```python
from build123d import *

# Parameters (mm, degrees)
SKETCH1_R           = 17
SKETCH1_R_2         = 8
BOSS_EXTRUDE4_DEPTH = 2
REVOLVE2_ANGLE      = 40
CIRPATTERN1_COUNT   = 3
FILLET1_R           = 5
BOSS_EXTRUDE6_DEPTH = 13
FILLET2_R           = 0.25
SKETCH25_R          = 0.9
CUT_EXTRUDE1_DEPTH  = 34.719430639
SKETCH26_R          = 1.55
CUT_EXTRUDE2_DEPTH  = 0.8


with BuildPart() as part:
    # Sketch1 → Boss-Extrude4 (new body)
    with BuildSketch(Plane(origin=(0, 0, 0), x_dir=(1, 0, 0), z_dir=(0, 1, 0))):
        with Locations(Location((0, 0, 0), (0, 0, 270))):
            Circle(SKETCH1_R)
        with Locations(Location((0, 0, 0), (0, 0, 270))):
            Circle(SKETCH1_R_2, mode=Mode.SUBTRACT)
    extrude(amount=BOSS_EXTRUDE4_DEPTH)

    # Sketch5 → Revolve2 (revolve)
    with BuildSketch(Plane.XY):
        Polygon((-17, 0), (-22, 0), (-21, 14), (-17, 14), align=None)
    revolve2 = revolve(axis=Axis((0, 9.813682869, 0), (0, -1, 0)), revolution_arc=REVOLVE2_ANGLE)

    # CirPattern1: Revolve2 ×3 about axis
    cirpattern1_axis = Axis((0, 0, 0), (0, 1, 0))
    for i in range(1, CIRPATTERN1_COUNT):
        add(revolve2.rotate(cirpattern1_axis, i * 360 / CIRPATTERN1_COUNT))

    # Fillet1
    fillet1_edges = [part.edges().sort_by_distance(p)[0] for p in [
        (-13.022755533, 1, -10.927389365),
        (-17, 1, 0),
        (-2.95201902, 1, 16.741731801),
        (8.5, 1, 14.722431864),
        (15.974774553, 1, -5.814342437),
        (8.5, 1, -14.722431864),
    ]]
    fillet(fillet1_edges, radius=FILLET1_R)

    # Sketch24 → Boss-Extrude6 (add)
    with BuildSketch(Plane(origin=(0, 2, 0), x_dir=(1, 0, 0), z_dir=(0, 1, 0))):
        with BuildLine():
            ThreePointArc((12.528097784, 11.491160338), (12.448209945, 10.445288373), (13.492065142, 10.342348776))
            ThreePointArc((13.492065142, 10.342348776), (13.022755533, 10.927389365), (12.528097784, 11.491160338))
        make_face()
    extrude(amount=BOSS_EXTRUDE6_DEPTH)

    # Fillet2
    # the kernel refuses this fillet: 0.25 mm, written as the material it takes off along each edge
    with BuildSketch(Plane(origin=(0, 15, 0), x_dir=(0.8154762444384231, 0, -0.578790544805809), z_dir=(0.578790544805809, 0, 0.8154762444384231))) as fillet2_piece_1:
        with BuildLine():
            CenterArc((17 - FILLET2_R, -FILLET2_R), FILLET2_R, 0, 90)
            Line((17 - FILLET2_R, 0), (17, 0))
            Line((17, 0), (17, -FILLET2_R))
        make_face()
    revolve(axis=Axis((0, 15, 0), (0, 1, 0)), revolution_arc=9.268958216, mode=Mode.SUBTRACT)

    # Sketch25 → Cut-Extrude1 (cut, through all)
    with BuildSketch(Plane(origin=(0, 2, 0), x_dir=(1, 0, 0), z_dir=(0, 1, 0))):
        with Locations(Location((2.083778132, -11.817693036, 0), (0, 0, 270))):
            Circle(SKETCH25_R)
        with Locations(Location((-11.236091343, 4.089602798, 0), (0, 0, 270))):
            Circle(SKETCH25_R)
        with Locations(Location((9.192533317, 7.713451316, 0), (0, 0, 270))):
            Circle(SKETCH25_R)
    extrude(amount=-CUT_EXTRUDE1_DEPTH, mode=Mode.SUBTRACT)

    # Sketch26 → Cut-Extrude2 (cut)
    with BuildSketch(Plane(origin=(0, 2, 0), x_dir=(1, 0, 0), z_dir=(0, 1, 0))):
        with Locations(Location((2.083778132, -11.817693036, 0), (0, 0, 270))):
            Circle(SKETCH26_R)
        with Locations(Location((-11.236091343, 4.089602798, 0), (0, 0, 270))):
            Circle(SKETCH26_R)
        with Locations(Location((9.192533317, 7.713451316, 0), (0, 0, 270))):
            Circle(SKETCH26_R)
    extrude(amount=-CUT_EXTRUDE2_DEPTH, mode=Mode.SUBTRACT)


solid = part.part
```
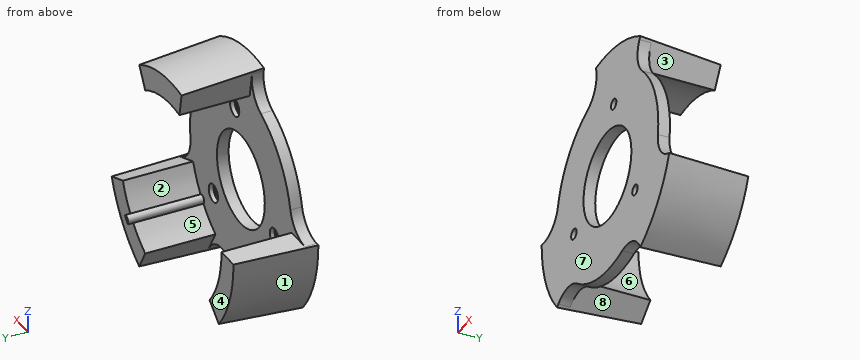
Geometry check sheet. Reference: the model listing, model coordinates, mm. Face numbers are marked on the shaded views. A direction names the side the tool comes from. Coordinates: 2 decimals unless noted, no trailing zeros. Loops run counter-clockwise (first coordinate to the right, second up) from the corner with the lowest first, then second, coordinate; pieces in that order, holes last. Notation, with made-up numbers: (-22, 42.5) - (4, 42.5) arc R16 cw to (4, 66.5) - close; hole circle Ø2 at (-11.5, 32.5). An arc over 180 degrees is marked (long way). One line per item, written item: value. Start each with the question number.
(1) Cross-section at D-D on y = 4. Enter the section's corners in (x, z).
(2) Mould release check, pull along Z, two halves, no side actions. Record for the marked faces 1, 2, 3 and 4: released by +Z, released by -Z, zero draft, split by the parting line, or undercut.
(3) Tool access check on the marked faces 5, 6, 7 and 8. Record the directions out of +Z, -Z, +X, -X, +Y, -Y that give a thin tool (end or side, any length) a straight path to the whole face; none if there is none.
(4) Material ranges on line 1 (Z direction, x = 1, y = 1.5); line 2 (Y direction, x = -8, z = -12.5); line 3 (Y direction, x = 18.5, z = -9.5), recorded low to high. Write a range as [from, to].
(5) Cross-section at B-B on y = 10.75. Enter the section's corners in (x, z).
(6) Cross-section at A-A on x = 0. Enter the section's corners in (y, z).
(7) Depth check by flat-ended pin: P1, Ø5, axis at x = 1.5, y = 8.5, coming from the -Z side; P2, Ø3, axis at x = 2, z = 17, coming from the +Y side; P3, Ø4, axis at x = -10, z = 16, coming from the +Y side. Enter the tip coordinate at first touch or a pass-through.
(8) Cross-section at C-C on x = -15.5. Enter the section's corners in (y, z).
Results below:
1. outline: (-21.71, 0) arc R21.71 ccw to (-16.63, -13.96) - (-13.02, -10.93) arc R17 cw to (-17, 0) - close; (-3.77, 21.38) - (-2.95, 16.74) arc R17 cw to (8.5, 14.72) - (10.86, 18.81) arc R21.71 ccw to start; (8.5, -14.72) - (10.86, -18.81) arc R21.71 ccw to (20.4, -7.43) - (15.97, -5.81) arc R17 cw to (13.49, -10.34) arc R0.75 ccw to (12.53, -11.49) arc R17 cw to start
2. face 1: released by -Z
2. face 2: released by +Z
2. face 3: undercut
2. face 4: zero draft
3. face 5: +Y
3. face 6: +Z, +Y
3. face 7: +Z, -Z, +X, -X, -Y
3. face 8: -Z, +Y
4. line 1: z = [-16.97, -7.94], [7.94, 10.71], [12.93, 21.87]
4. line 2: y = [0, 2]
4. line 3: y = [0, 14]
5. outline: (-21.23, 0) arc R21.23 ccw to (-16.26, -13.65) - (-13.02, -10.93) arc R17 cw to (-17, 0) - close; (-3.69, 20.91) - (-2.95, 16.74) arc R17 cw to (8.5, 14.72) - (10.62, 18.39) arc R21.23 ccw to start; (8.5, -14.72) - (10.62, -18.39) arc R21.23 ccw to (19.95, -7.26) - (15.97, -5.81) arc R17 cw to (13.49, -10.34) arc R0.75 ccw to (12.53, -11.49) arc R17 cw to start
6. outline: (0, -17) - (2, -17) - (2, -8) - (0, -8) - close; (0, 8) - (2, 8) - (2, 17) - (14, 17) - (14, 21) - (0, 22) - close
7. P1: stops at z = 16.52
7. P2: stops at y = 14
7. P3: stops at y = 2
8. outline: (0, -13.16) - (2, -13.16) - (2, -13.01) - (14, -13.01) - (14, -6.98) - (2, -6.98) - (2, 6.98) - (0, 6.98) - close
